CAD build for the part. Positions are in the model's coordinates, mm. A direction names the side the tool comes from. Coordinates: 2 decimals unless noted, no trailing zeros. Loops run counter-clockwise (first coordinate to the right, second up) from the corner with the lowest first, then second, coordinate; pieces in that order, holes last. Notation, with made-up numbers: (-30.75, 5) - (-23.75, 5) arc R12 cw to (-23.75, 26) - close; hole circle Ø9 at (33.5, -38.5). An arc over 180 degrees is marked (long way). Put each result on its own line as item: value.
```python
from build123d import *

# Parameters (mm, degrees)
SKETCH2_W           = 736.6
SKETCH2_H           = 38.1
BOSS_EXTRUDE1_DEPTH = 12.7
SKETCH3_W           = 38.1
SKETCH3_H           = 38.1
BOSS_EXTRUDE2_DEPTH = 431.8
SKETCH4_R           = 6.35
CUT_EXTRUDE1_DEPTH  = 737.6


with BuildPart() as part:
    # Sketch2 → Boss-Extrude1 (new body)
    with BuildSketch(Plane(origin=(0, 0, 0), x_dir=(1, 0, 0), z_dir=(0, 1, 0))):
        Rectangle(SKETCH2_W, SKETCH2_H)
    extrude(amount=BOSS_EXTRUDE1_DEPTH)

    # Sketch3 → Boss-Extrude2 (add)
    with BuildSketch(Plane(origin=(0, 12.7, 0), x_dir=(1, 0, 0), z_dir=(0, 1, 0))):
        with Locations((-349.25, 0)):
            Rectangle(SKETCH3_W, SKETCH3_H)
        with Locations((349.25, 0)):
            Rectangle(SKETCH3_W, SKETCH3_H)
    extrude(amount=BOSS_EXTRUDE2_DEPTH)

    # Sketch4 → Cut-Extrude1 (cut, through all)
    with BuildSketch(Plane(origin=(368.3, 0, 0), x_dir=(0, 0, -1), z_dir=(1, 0, 0))):
        with Locations((0, 419.1)):
            Circle(SKETCH4_R)
    extrude(amount=-CUT_EXTRUDE1_DEPTH, mode=Mode.SUBTRACT)


solid = part.part
```
Q1. Slice it at A-A, the plane z = 0. Give the cut face in (x, y).
Determined:
outline: (-368.3, 0) - (368.3, 0) - (368.3, 412.75) - (330.2, 412.75) - (330.2, 12.7) - (-330.2, 12.7) - (-330.2, 412.75) - (-368.3, 412.75) - close; (-368.3, 425.45) - (-330.2, 425.45) - (-330.2, 444.5) - (-368.3, 444.5) - close; (330.2, 425.45) - (368.3, 425.45) - (368.3, 444.5) - (330.2, 444.5) - close
Q2. Wall check: L1, parallel to X at y = 196, z = -14; L2, parallel to Y at x = 358.5, z = 0; L3, parallel to Z at x = -341, y = 419. Give the ranges that are in metal, low to high. Write a range as from..to.
Determined:
L1: -368.3..-330.2, 330.2..368.3
L2: 0..412.75, 425.45..444.5
L3: -19.05..-6.35, 6.35..19.05
Q3. Slice it at C-C, the plane x = 12.5. Give the cut face in (y, z).
Determined:
outline: (0, -19.05) - (12.7, -19.05) - (12.7, 19.05) - (0, 19.05) - close
Q4. Mould opens along X. For faces 3 (the flat face through (-330.2, 226, 0)), 4 (the flat face through (-368.3, 219, 0)), 5 (the flat face through (-5, 0, 0)) say: +X half, -X half, draft (parallel to the pull), parting line (faces both ways), or undercut.
Determined:
face 3: undercut
face 4: -X half
face 5: draft
Q5. Pin check, flat tips, straight feed: pin 1 Ø2 at (x, z) = (-115, -12.5) entering from +Y; pin 2 Ø10 at (y, z) = (419.1, 0) entering from +X. Stop position of each tip, or through.
Determined:
pin 1: y = 12.7
pin 2: through
Q6. Tool access for faces 1 (the flat face through (330.2, 226, 0)), 2 (the flat face through (368.3, 219, 0)): list every direction of +Z, -Z, +X, -X, +Y, -Y with a clear straight run to the whole face (end or side of a thin tool).
Determined:
face 1: +Z, -Z, +Y
face 2: +Z, -Z, +X, +Y, -Y
Q7. Slice it at B-B, the plane y = 141. Give the cut face in (x, z), then the cut area to 3 significant figures.
Determined:
outline: (-368.3, -19.05) - (-330.2, -19.05) - (-330.2, 19.05) - (-368.3, 19.05) - close; (330.2, -19.05) - (368.3, -19.05) - (368.3, 19.05) - (330.2, 19.05) - close
area: 2,900 mm2
